Read the model definition and answer for the solid it produces. Units are mm, in the model's axes. A direction names the side the tool comes from. Coordinates: 2 decimals unless noted, no trailing zeros. Loops run counter-clockwise (first coordinate to the right, second up) from the corner with the lowest first, then second, coordinate; pieces in that order, holes last. Notation, with made-up numbers: (6, 31) -> (41, 31) arc R5 ccw to (41, 35) -> close; hole circle Ø9 at (-35, 79). An arc over 180 degrees is marked (long way). Answer in a Markdown table with one row per item.
```python
from build123d import *

# Parameters (mm, degrees)
F1_DEPTH = 63.5
F2_DEPTH = 25.4
F3_DEPTH = 7.9375
F4_DEPTH = 25.4
F5_R     = 6.35


with BuildPart() as f1:
    # F0 (on Front) → F1 (new body, symmetric)
    with BuildSketch(Plane.XZ):
        Polygon((-41.275, -9.525), (41.275, -9.525), (41.275, 9.525), (22.225, 9.525), (-41.275, 9.525), align=None)
    extrude(amount=F1_DEPTH, both=True)

    # F0 (on Front) → F2 (join, symmetric)
    with BuildSketch(Plane.XZ):
        with BuildLine():
            Line((22.225, 9.525), (41.275, 9.525))
            Line((41.275, 9.525), (41.275, 27.0002))
            ThreePointArc((41.275, 27.0002), (45.9246798487, 38.2255201513), (57.15, 42.8752))
            Line((57.15, 42.8752), (60.325, 42.8752))
            Line((60.325, 42.8752), (60.325, 61.9252))
            Line((60.325, 61.9252), (57.15, 61.9252))
            ThreePointArc((57.15, 61.9252), (32.4542956671, 51.6959043329), (22.225, 27.0002))
            Line((22.225, 27.0002), (22.225, 9.525))
        make_face()
    extrude(amount=F2_DEPTH, both=True)

    # F0 (on Front) → F3 (join, symmetric)
    with BuildSketch(Plane.XZ):
        with BuildLine():
            add(Edge.make_bspline(
                [(-41.275, 9.525), (-12.3398668578, 41.355177187), (20.8714975106, 60.4699858623), (60.325, 66.675)],
                knots=[0, 0, 0, 0, 116.5705044169, 116.5705044169, 116.5705044169, 116.5705044169], degree=3))
            Line((-41.275, 9.525), (22.225, 9.525))
            Line((22.225, 9.525), (22.225, 27.0002))
            ThreePointArc((22.225, 27.0002), (32.4542956671, 51.6959043329), (57.15, 61.9252))
            Line((57.15, 61.9252), (60.325, 61.9252))
            Line((60.325, 61.9252), (60.325, 66.675))
        make_face()
    extrude(amount=F3_DEPTH, both=True)

    # F0 (on Front) → F4 (join, symmetric)
    with BuildSketch(Plane.XZ):
        Polygon((92.7243528686, 61.9252), (60.325, 61.9252), (60.325, 42.8752), (60.325, 38.1), (92.6698073745, 38.1), align=None)
    extrude(amount=F4_DEPTH, both=True)

    # F5
    f5_edges = [f1.edges().sort_by_distance(p)[0] for p in [
        (-41.275, -63.5, 0),
        (41.275, -63.5, 0),
        (41.275, 63.5, 0),
        (-41.275, 63.5, 0),
    ]]
    fillet(f5_edges, radius=F5_R)

    # F0 (on Front) → F6 (revolve)
    with BuildSketch(Plane.XZ):
        Polygon((111.125, 66.675), (92.7352270769, 66.675), (92.7243528686, 61.9252), (92.6698073745, 38.1), (111.125, 38.1), align=None)
    revolve(axis=Axis((92.7025172257, 0, 52.3875), (0.0022893974, 0, 0.9999973793)))


solid = f1.part
```
1. A cutting plane is placed at A-A on y = -20.5. Give the vertices of the cut face in (x, z) (3 decimals).
A:
| item | result |
|---|---|
| outline | (-41.275, -9.525) -> (41.275, -9.525) -> (41.275, 27) arc R15.875 cw to (57.15, 42.875) -> (60.325, 42.875) -> (60.325, 38.1) -> (92.67, 38.1) -> (92.724, 61.925) -> (57.15, 61.925) arc R34.925 ccw to (22.225, 27) -> (22.225, 9.525) -> (-41.275, 9.525) -> close |
2. A cutting plane is placed at B-B on y = -34.5. Give the vertices of the cut face in (x, z) (3 decimals).
A:
| item | result |
|---|---|
| outline | (-41.275, -9.525) -> (41.275, -9.525) -> (41.275, 9.525) -> (-41.275, 9.525) -> close |
3. A tool of negligible diameter and unlimited length cuts with its end or side. For faces 4 (the flat face through (22.225, 17, 18)), 5 (the flat face through (41.275, -1, 4)), 6 (the flat face through (60.325, 0, 41)), from which of +Z, -Z, +X, -X, +Y, -Y can it reach the whole face along a straight path? Write none if from no direction.
A:
| item | result |
|---|---|
| face 4 | +Z, -X, +Y |
| face 5 | -Z, +X, +Y, -Y |
| face 6 | -Z, +Y, -Y |
4. The mould has two halves that part along X. Classify faces 1 (the cylindrical face through (45.8, -0.4, 38.1)), 2 (the flat face through (76, 0, 38.1)), 3 (the flat face through (22.225, -17, 18)): pulls with the +X half, pulls with the -X half, needs draft (parallel to the pull), parting line crosses it, or undercut.
A:
| item | result |
|---|---|
| face 1 | undercut |
| face 2 | needs draft |
| face 3 | pulls with the -X half |
5. Given pin 1 Ø8 at (x, z) = (-11.5, 44.5) entering from +Y; pin 2 Ø2 at (x, y) = (64.5, -15) entering from +Z; pin 3 Ø16 at (x, y) = (72, -1) entering from -Z; pin 4 Ø1.6 at (x, y) = (59, 11.5) entering from -Z, each flat-ended and moving along its own axis, determine where each tip first touches the part or whether it passes through.
A:
| item | result |
|---|---|
| pin 1 | passes through |
| pin 2 | stops at z = 61.93 |
| pin 3 | stops at z = 38.1 |
| pin 4 | stops at z = 42.88 |
6. Find the intervals of material crossed by probe 1 along Y at (x, z) = (8, 29.5); probe 2 along Z at (x, y) = (76, 0.5); probe 3 along Z at (x, y) = (3, -14) (3 decimals), in increasing order.
A:
| item | result |
|---|---|
| probe 1 | y = -7.94 to 7.94 |
| probe 2 | z = 38.1 to 66.75 |
| probe 3 | z = -9.525 to 9.525 |
